from build123d import *

# Parameters (mm, degrees)
F0_R     = 6.35
F1_DEPTH = 19.05
F2_R     = 35.17899


# Not quite as in the source:
# - a fillet or chamfer is up to 0.001 mm smaller than in the source, because OpenCascade refuses the exact size


with BuildPart() as f1:
    # F0 (on Top) → F1 (new body)
    with BuildSketch(Plane.XY):
        with BuildLine():
            Line((372.999, 22.479), (-48.26, 22.479))
            ThreePointArc((-48.26, 22.479), (-83.439, -12.7), (-48.26, -47.879))
            Line((-48.26, -47.879), (372.999, -47.879))
            Line((372.999, -47.879), (372.999, 22.479))
        make_face()
        Circle(F0_R, mode=Mode.SUBTRACT)
        with Locations((276.225, -12.7)):
            Circle(F0_R, mode=Mode.SUBTRACT)
    extrude(amount=F1_DEPTH)

    # F2 (radius 35.179 in the source; OpenCascade refuses exactly that, so slightly less here)
    f2_edges = [f1.edges().sort_by_distance(p)[0] for p in [
        (372.999, -47.879, 9.525),
        (372.999, 22.479, 9.525),
    ]]
    fillet(f2_edges, radius=F2_R)


solid = f1.part
Model file for the job. Use its own axes, mm. Coordinates: 2 decimals unless noted, no trailing zeros. Order: outer loops, then holes, each group sorted by start corner. A loop starts at its lowest first (then second) coordinate and runs counter-clockwise, first axis right, second up. Notation, with made-up numbers: M 9.25,28 L 36.25,28 A30 ccw 36.25,55 Z; hole C 61,11.5 d3. An arc over 180 degrees is marked long. Return JSON: item names as keys, results as strings.
1. Drill centre lines: probe 1 along Y at (x, z) = (0, 5); probe 2 along X at (y, z) = (-14.5, 11); probe 3 along Y at (x, z) = (4, 9). Where is each one in solid material? Low to high.
Ans:
{"probe 1": "-47.88 to -6.35, 6.35 to 22.48", "probe 2": "-83.39 to 270.14, 282.31 to 372.95", "probe 3": "-47.88 to -4.93, 4.93 to 22.48"}
2. Saw through at D-D (y = -33). Give the cut face in (x, z), and give its area (3 significant figures).
Ans:
{"outline": "M -76.99,0 L 366.55,0 L 366.55,19.05 L -76.99,19.05 Z", "area": "8,450 mm^2"}
3. Flat gauge pins, fed straight in: pin 1 (4 mm diameter, centred on x = 150.5, y = -27, fed in from -Z); pin 2 (3 mm diameter, centred on y = -10, z = 5, fed in from -X); pin 3 (6 mm diameter, centred on y = -34, z = 11, fed in from +X). Where does each tip first touch, or does it go through?
Ans:
{"pin 1": "z = 0", "pin 2": "x = -83.42", "pin 3": "x = 367.86"}
4. Saw through at B-B (x = 0). Give the cut face in (y, z), and give its area (3 significant figures).
Ans:
{"outline": "M -47.88,0 L -6.35,0 L -6.35,19.05 L -47.88,19.05 Z; M 6.35,0 L 22.48,0 L 22.48,19.05 L 6.35,19.05 Z", "area": "1,100 mm^2"}
5. Saw through at C-C (y = 0). Give the cut face in (x, z).
Ans:
{"outline": "M -81.07,0 L -6.35,0 L -6.35,19.05 L -81.07,19.05 Z; M 6.35,0 L 370.63,0 L 370.63,19.05 L 6.35,19.05 Z"}
6. Pull direction X, two halves, no side cores. Call faces 1 (the face through (362.42, 12.45, 9.66)), 2 (the face through (-1.38, -6.2, 9.39)), 3 (the face through (-83.43, -11.93, 9.39)): +X half, -X half, draft (parallel to the pull), parting line (faces both ways), or undercut.
Ans:
{"face 1": "+X half", "face 2": "undercut", "face 3": "-X half"}
7. Saw through at A-A (z = 3.75). Give the number of separate pieces and of enclosed holes in the cut face, and give its area (3 significant figures).
Ans:
{"separate pieces": "1", "enclosed holes": "2", "area": "30,800 mm^2"}
